Geometry check sheet. Reference: the model listing, model coordinates, mm. A direction names the side the tool comes from. Round coordinates to 2 decimals unless told otherwise and drop trailing zeros. Order: outer loops, then holes, each group sorted by start corner. A loop starts at its lowest first (then second) coordinate and runs counter-clockwise, first axis right, second up.
(1) Draft check along X on faces 1 (the face through (-14.605, 4.94, -6.132)), 2 (the face through (-13.908, 5.06, -5.895)), 3 (the face through (0, 5, 90.801)). Enter one of: pulls with the +X half, pulls with the -X half, needs draft (parallel to the pull), parting line crosses it, or undercut.
(2) Cross-section at A-A on y = 7.5. Enter the section's corners in (x, z).
(3) Cross-section at B-B on x = 18.5. Enter the section's corners in (y, z).
(4) Cross-section at C-C on x = 31. Enter the section's corners in (y, z).
(5) Set-up check for faces 4 (the face through (0, 5, 90.065)), 5 (the face through (10, 0, 18)), 6 (the face through (-14.2, -0.3, -6)), 7 (the face through (40.541, 5, 1)): record each of +Z, -Z, +X, -X, +Y, -Y from which the full face is reachable in a straight line by a thin tool's end or side.
(6) Gauge pin test, flat ends, axial feed: P1, Ø3, axis at x = 27.5, y = 7.5, coming from the -Z side; P2, Ø1, axis at x = -5.5, z = 45, coming from the +Y side; P3, Ø0.6, axis at x = 40.5, y = 5, coming from the -Z side; P4, Ø5, axis at y = 6, z = 42.5, coming from the -X side. Record the tip position at first contact, or that the pin passes through.
(7) Thickness scan on L1, parallel to X at y = 0.25, z = -7.5; L2, parallel to Y at x = 32, z = -56; L3, parallel to X at y = 8, z = 5. Record the ranges inside material, lowest first.
from build123d import *

# Parameters (mm, degrees)
BASE_FLANGE1_DEPTH            = 0.7366
EDGE_FLANGE1_STRIP_W          = 4.4196
EDGE_FLANGE1_STRIP_H          = 0.7366
EDGE_FLANGE1_STRIP_CUT_DEPTH  = 150
EDGE_FLANGE1_RELIEF_W         = 4.7879
EDGE_FLANGE1_RELIEF_H         = 0.3683
EDGE_FLANGE1_RELIEF_CUT_DEPTH = 0.7366
EDGE_FLANGE1_DEPTH            = 150
EDGE_FLANGE2_STRIP_W          = 4.4196
EDGE_FLANGE2_STRIP_H          = 0.7366
EDGE_FLANGE2_STRIP_CUT_DEPTH  = 50.953389831
EDGE_FLANGE2_RELIEF_W         = 4.7879
EDGE_FLANGE2_RELIEF_H         = 0.3683
EDGE_FLANGE2_RELIEF_CUT_DEPTH = 0.7366
EDGE_FLANGE2_DEPTH            = 50.953389831
EDGE_FLANGE3_STRIP_W          = 4.4196
EDGE_FLANGE3_STRIP_H          = 0.7366
EDGE_FLANGE3_STRIP_CUT_DEPTH  = 158.417953324
EDGE_FLANGE3_RELIEF_W         = 4.7879
EDGE_FLANGE3_RELIEF_H         = 0.3683
EDGE_FLANGE3_RELIEF_CUT_DEPTH = 0.7366
EDGE_FLANGE3_DEPTH            = 158.417953324


# Sheet-metal steps are written as plain solids
with BuildPart() as part:
    # Sketch1 → Base-Flange1 (new body)
    with BuildSketch(Plane(origin=(0, 0, 0), x_dir=(1, 0, 0), z_dir=(0, 1, 0))):
        with BuildLine():
            Line((40.54139599, 75), (40.54139599, -75))
            ThreePointArc((40.54139599, -75), (36.129047202, -85.652352287), (25.476694915, -90.064701075))
            Line((25.476694915, -90.064701075), (-25.476694915, -90.064701075))
            ThreePointArc((-25.476694915, -90.064701075), (-37.722911645, -83.773562235), (-39.740893599, -70.154604826))
            Line((-39.740893599, -70.154604826), (11.212496231, 79.845395174))
            ThreePointArc((11.212496231, 79.845395174), (28.299643698, 92.087147467), (40.54139599, 75))
        make_face()
    extrude(amount=-BASE_FLANGE1_DEPTH)

    # Edge-Flange1 strip (across the edge) → Edge-Flange1 strip cut (cut)
    with BuildSketch(Plane(origin=(40.54139599, 0, 75), x_dir=(-1, 0, 0), z_dir=(0, 0, -1))):
        with Locations((-1.4732, -0.3683)):
            Rectangle(EDGE_FLANGE1_STRIP_W, EDGE_FLANGE1_STRIP_H)
    extrude(amount=EDGE_FLANGE1_STRIP_CUT_DEPTH, mode=Mode.SUBTRACT)

    # Edge-Flange1 relief (on the sheet) → Edge-Flange1 relief cut (cut)
    with BuildSketch(Plane(origin=(39.80479599, 0, 75), x_dir=(-1, 0, 0), z_dir=(0, 1, 0))):
        with Locations((-2.02565, 0.18415)):
            Rectangle(EDGE_FLANGE1_RELIEF_W, EDGE_FLANGE1_RELIEF_H)
        with Locations((-2.02565, -150.18415)):
            Rectangle(EDGE_FLANGE1_RELIEF_W, EDGE_FLANGE1_RELIEF_H)
    extrude(amount=-EDGE_FLANGE1_RELIEF_CUT_DEPTH, mode=Mode.SUBTRACT)

    # Edge-Flange1 section (across the edge) → Edge-Flange1 (add)
    with BuildSketch(Plane(origin=(40.54139599, 0, 75), x_dir=(-1, 0, 0), z_dir=(0, 0, -1))):
        with BuildLine():
            Line((-0.7366, 0.7366), (-0.7366, 9.2634))
            Line((-0.7366, 9.2634), (0, 9.2634))
            Line((0, 9.2634), (0, 0.7366))
            ThreePointArc((0, 0.7366), (0.215745145, 0.215745145), (0.7366, 0))
            Line((0.7366, 0), (0.7366, -0.7366))
            ThreePointArc((0.7366, -0.7366), (-0.30510971, -0.30510971), (-0.7366, 0.7366))
        make_face()
    extrude(amount=EDGE_FLANGE1_DEPTH)

    # Edge-Flange2 strip (across the edge) → Edge-Flange2 strip cut (cut)
    with BuildSketch(Plane(origin=(-25.476694915, 0, 90.064701075), x_dir=(0, 0, -1), z_dir=(1, 0, 0))):
        with Locations((-1.4732, -0.3683)):
            Rectangle(EDGE_FLANGE2_STRIP_W, EDGE_FLANGE2_STRIP_H)
    extrude(amount=EDGE_FLANGE2_STRIP_CUT_DEPTH, mode=Mode.SUBTRACT)

    # Edge-Flange2 relief (on the sheet) → Edge-Flange2 relief cut (cut)
    with BuildSketch(Plane(origin=(-25.476694915, 0, 89.328101075), x_dir=(0, 0, -1), z_dir=(0, 1, 0))):
        with Locations((-2.02565, 0.18415)):
            Rectangle(EDGE_FLANGE2_RELIEF_W, EDGE_FLANGE2_RELIEF_H)
        with Locations((-2.02565, -51.137539831)):
            Rectangle(EDGE_FLANGE2_RELIEF_W, EDGE_FLANGE2_RELIEF_H)
    extrude(amount=-EDGE_FLANGE2_RELIEF_CUT_DEPTH, mode=Mode.SUBTRACT)

    # Edge-Flange2 section (across the edge) → Edge-Flange2 (add)
    with BuildSketch(Plane(origin=(-25.476694915, 0, 90.064701075), x_dir=(0, 0, -1), z_dir=(1, 0, 0))):
        with BuildLine():
            Line((-0.7366, 0.7366), (-0.7366, 9.2634))
            Line((-0.7366, 9.2634), (0, 9.2634))
            Line((0, 9.2634), (0, 0.7366))
            ThreePointArc((0, 0.7366), (0.215745145, 0.215745145), (0.7366, 0))
            Line((0.7366, 0), (0.7366, -0.7366))
            ThreePointArc((0.7366, -0.7366), (-0.30510971, -0.30510971), (-0.7366, 0.7366))
        make_face()
    extrude(amount=EDGE_FLANGE2_DEPTH)

    # Edge-Flange3 strip (across the edge) → Edge-Flange3 strip cut (cut)
    with BuildSketch(Plane(origin=(11.212496231, 0, -79.845395174), x_dir=(0.9468623779885023, 3.4914813388431334e-15, 0.3216389857432692), z_dir=(-0.3216389857432692, 0, 0.9468623779885023))):
        with Locations((-1.4732, -0.3683)):
            Rectangle(EDGE_FLANGE3_STRIP_W, EDGE_FLANGE3_STRIP_H)
    extrude(amount=EDGE_FLANGE3_STRIP_CUT_DEPTH, mode=Mode.SUBTRACT)

    # Edge-Flange3 relief (on the sheet) → Edge-Flange3 relief cut (cut)
    with BuildSketch(Plane(origin=(11.909955059, 0, -79.608475897), x_dir=(0.9468623779885023, 6.982962677686267e-15, 0.3216389857432692), z_dir=(0, 1, 0))):
        with Locations((-2.02565, 0.18415)):
            Rectangle(EDGE_FLANGE3_RELIEF_W, EDGE_FLANGE3_RELIEF_H)
        with Locations((-2.02565, -158.602103324)):
            Rectangle(EDGE_FLANGE3_RELIEF_W, EDGE_FLANGE3_RELIEF_H)
    extrude(amount=-EDGE_FLANGE3_RELIEF_CUT_DEPTH, mode=Mode.SUBTRACT)

    # Edge-Flange3 section (across the edge) → Edge-Flange3 (add)
    with BuildSketch(Plane(origin=(11.212496231, 0, -79.845395174), x_dir=(0.9468623779885023, 3.4914813388431334e-15, 0.3216389857432692), z_dir=(-0.3216389857432692, 0, 0.9468623779885023))):
        with BuildLine():
            Line((-0.7366, 0.7366), (-0.7366, 9.2634))
            Line((-0.7366, 9.2634), (0, 9.2634))
            Line((0, 9.2634), (0, 0.7366))
            ThreePointArc((0, 0.7366), (0.215745145, 0.215745145), (0.7366, 0))
            Line((0.7366, 0), (0.7366, -0.7366))
            ThreePointArc((0.7366, -0.7366), (-0.30510971, -0.30510971), (-0.7366, 0.7366))
        make_face()
    extrude(amount=EDGE_FLANGE3_DEPTH)


solid = part.part
Found:
1. face 1: pulls with the -X half
1. face 2: undercut
1. face 3: needs draft
2. outline: (-40.44, 69.92) - (10.52, -80.08) - (11.21, -79.85) - (-39.74, 70.15) - close; (-25.48, 90.06) - (25.48, 90.06) - (25.48, 90.8) - (-25.48, 90.8) - close; (40.54, -75) - (41.28, -75) - (41.28, 75) - (40.54, 75) - close
3. outline: (-0.74, -90.33) - (0, -90.33) - (0, 89.33) arc R0.74 cw to (0.74, 90.06) - (9.26, 90.06) - (9.26, 90.8) - (0.74, 90.8) arc R1.47 ccw to (-0.74, 89.33) - close
4. outline: (-0.74, -91.38) - (0, -91.38) - (0, 89.02) - (-0.74, 89.02) - close
5. face 4: +X, -X, +Y
5. face 5: +Y
5. face 6: -Z, -X, -Y
5. face 7: +Z, -Z, +Y
6. P1: passes through
6. P2: stops at y = 0
6. P3: stops at z = -75
6. P4: stops at x = -31.97
7. L1: x = -14.05 to -13.17, 40.36 to 41.2
7. L2: y = -0.74 to 0
7. L3: x = -18.39 to -17.61, 40.54 to 41.28
